from build123d import *

# Parameters (mm, degrees)
SKETCH1_W           = 91.948
SKETCH1_H           = 76.2
BOSS_EXTRUDE1_DEPTH = 4.7625
BOSS_EXTRUDE2_START = -4.7625
SKETCH2_W           = 91.948
SKETCH2_H           = 44.45
BOSS_EXTRUDE2_DEPTH = 12.7
SKETCH3_R           = 10.3124
CUT_EXTRUDE6_DEPTH  = 125.421181191
SKETCH4_R           = 2.5527
CUT_EXTRUDE7_DEPTH  = 12.7


with BuildPart() as part:
    # Sketch1 → Boss-Extrude1 (new body)
    with BuildSketch(Plane.XY):
        with Locations((45.974, 38.1)):
            Rectangle(SKETCH1_W, SKETCH1_H)
    boss_extrude1 = extrude(amount=BOSS_EXTRUDE1_DEPTH)

    # Sketch2 → Boss-Extrude2 (add)
    with BuildSketch(Plane(origin=(0, 0, 0), x_dir=(-1, 0, 0), z_dir=(0, 0, -1)).offset(BOSS_EXTRUDE2_START)):
        with Locations((-45.974, 38.1)):
            Rectangle(SKETCH2_W, SKETCH2_H)
    boss_extrude2 = extrude(amount=-BOSS_EXTRUDE2_DEPTH)

    # Mirror1: Boss-Extrude1, Boss-Extrude2 across plane
    add(boss_extrude1.mirror(Plane.XY))
    add(boss_extrude2.mirror(Plane.XY))

    # Sketch3 → Cut-Extrude6 (cut, through all)
    with BuildSketch(Plane.XY.offset(17.4625)):
        with Locations((25.4, 38.1)):
            Circle(SKETCH3_R)
        with Locations((65.786, 38.1)):
            Circle(SKETCH3_R)
    extrude(amount=-CUT_EXTRUDE6_DEPTH, mode=Mode.SUBTRACT)

    # Sketch4 → Cut-Extrude7 (cut)
    with BuildSketch(Plane.XY.offset(17.4625)):
        with Locations((6.35, 50.8)):
            Circle(SKETCH4_R)
        with Locations((6.35, 25.4)):
            Circle(SKETCH4_R)
        with Locations((45.974, 25.4)):
            Circle(SKETCH4_R)
        with Locations((45.974, 50.8)):
            Circle(SKETCH4_R)
        with Locations((85.598, 50.8)):
            Circle(SKETCH4_R)
        with Locations((85.598, 25.4)):
            Circle(SKETCH4_R)
    extrude(amount=-CUT_EXTRUDE7_DEPTH, mode=Mode.SUBTRACT)


solid = part.part
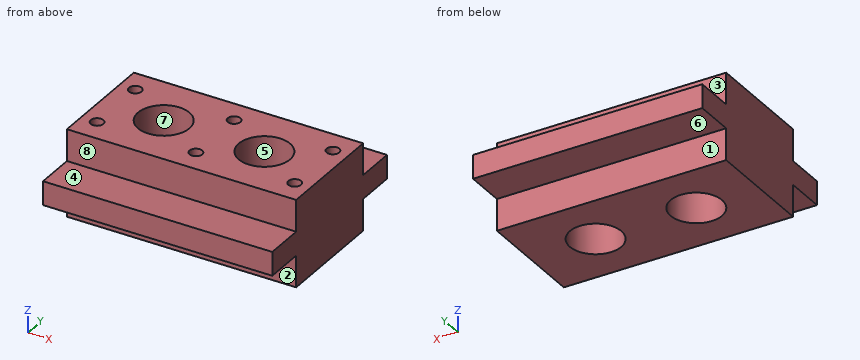
The model under review builds one solid part; all positions refer to its coordinate system, in mm. Face numbers are marked on the shaded views. A direction names the side the tool comes from. Coordinates: 2 decimals unless noted, no trailing zeros. Loops run counter-clockwise (first coordinate to the right, second up) from the corner with the lowest first, then second, coordinate; pieces in that order, holes last. Notation, with made-up numbers: (6, -10.5) -> (20, -10.5) arc R33 cw to (20, 25.5) -> close; hole circle Ø10 at (-24.75, 67.25). An arc over 180 degrees is marked (long way). Use a Markdown table: item, result. Add a question column.
1. Machinability: for the marked faces 1, 2, 3 and 4, which of the approach directions +Z, -Z, +X, -X, +Y, -Y give a long, thin tool a straight path to every point of the face, cutting with its end or side? Answer none if there is none.
2. Add section B-B on y = 38.1. Write out the cut boundary in (x, z).
3. Draft analysis for pull direction Y (two halves, no side actions). For the marked faces 5, 6, 7 and 8, state which applies: pulls with the +Y half, pulls with the -Y half, needs draft (parallel to the pull), parting line crosses it, or undercut.
4. Add section D-D on z = -14.5. Write out the cut boundary in (x, y) (3 decimals), plus the area to 3 significant figures.
5. Clearance check with flat-ended pins moving along their axes: pin 1 Ø1 at (x, z) = (66, -10.5) entering from -Y (3 decimals); pin 2 Ø1.5 at (x, y) = (85, 26) entering from +Z; pin 3 Ø17.5 at (x, y) = (63, 72) entering from -Z. State where each tip first meets the part, or that it passes through.
6. Add section C-C on z = 6.5. Give the number of separate pieces and of enclosed holes in the cut face, plus the area to 3 significant figures.
7. To check wall thickness, follow line 1 (Y direction, x = 6, z = 6) (3 decimals); line 2 (X direction, y = 38, z = 0); line 3 (Y direction, x = 6.35, z = 14.75) (3 decimals). State the ranges of each line that lie inside material, in increasing order.
8. Add section A-A on x = 25.4. Write out the cut boundary in (y, z) (1 decimal), plus the area to 3 significant figures.
Returned:
| question | item | result |
|---|---|---|
| 1 | face 1 | -Z, +X, -X, +Y |
| 1 | face 2 | -Z, +X, -X, -Y |
| 1 | face 3 | +Z, +X, -X, +Y |
| 1 | face 4 | +Z, +X, -X, -Y |
| 2 | outline | (0, -17.46) -> (15.09, -17.46) -> (15.09, 17.46) -> (0, 17.46) -> close; (35.71, -17.46) -> (55.47, -17.46) -> (55.47, 17.46) -> (35.71, 17.46) -> close; (76.1, -17.46) -> (91.95, -17.46) -> (91.95, 17.46) -> (76.1, 17.46) -> close |
| 3 | face 5 | undercut |
| 3 | face 6 | needs draft |
| 3 | face 7 | undercut |
| 3 | face 8 | pulls with the -Y half |
| 4 | outline | (0, 15.875) -> (91.948, 15.875) -> (91.948, 60.325) -> (0, 60.325) -> close; hole circle Ø20.625 at (25.4, 38.1); hole circle Ø20.625 at (65.786, 38.1) |
| 4 | area | 3,420 mm² |
| 5 | pin 1 | stops at y = 15.875 |
| 5 | pin 2 | stops at z = 4.76 |
| 5 | pin 3 | stops at z = -4.76 |
| 6 | separate pieces | 1 |
| 6 | enclosed holes | 8 |
| 6 | area | 3,300 mm² |
| 7 | line 1 | y = 15.875 to 22.871, 27.929 to 48.271, 53.329 to 60.325 |
| 7 | line 2 | x = 0 to 15.09, 35.71 to 55.47, 76.1 to 91.95 |
| 7 | line 3 | y = 15.875 to 22.847, 27.953 to 48.247, 53.353 to 60.325 |
| 8 | outline | (0, -4.8) -> (15.9, -4.8) -> (15.9, -17.5) -> (27.8, -17.5) -> (27.8, 17.5) -> (15.9, 17.5) -> (15.9, 4.8) -> (0, 4.8) -> close; (48.4, -17.5) -> (60.3, -17.5) -> (60.3, -4.8) -> (76.2, -4.8) -> (76.2, 4.8) -> (60.3, 4.8) -> (60.3, 17.5) -> (48.4, 17.5) -> close |
| 8 | area | 1,130 mm² |
